Can you work these out from the drawing? Everything is in mm from the part's minimum corner. Coordinates: 2 decimals unless noted, no trailing zeros. Order: outer loops, then holes, each group sorted by start corner. A loop starts at its lowest first (then second) coordinate and runs counter-clockwise, first axis right, second up. Notation, with made-up numbers: M 83.25,84.5 L 115.25,84.5 A20 ccw 115.25,108.5 Z; hole C 68,13.5 d4. An arc over 180 degrees is marked long. Answer as CSV lines item,"result". Start each with the question number.
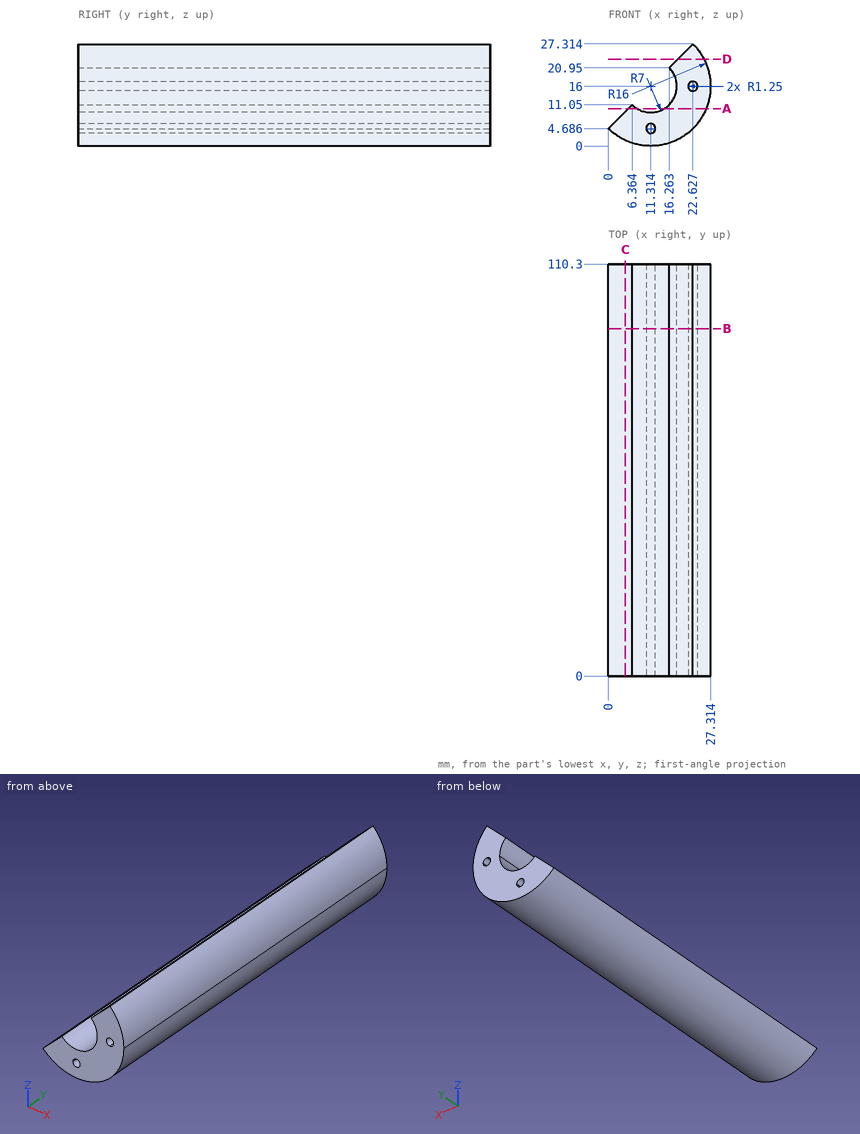
1) Suppose I cut it at D-D on z = 23.25. Please give me the cut outline in (x, y).
2) Suppose I cut it at A-A on z = 10. Please give me the cut outline in (x, y), plus the area to 3 significant figures.
3) Suppose I cut it at B-B on y = 93. Give the number of separate pieces and of enclosed holes in the cut face, plus the area to 3 significant figures.
4) Will these pins go through, and if not, where does the flat tip stop? pin 1 Ø12 at (x, z) = (23, 12) entering from -Y; pin 2 Ø12 at (x, y) = (18.5, 93) entering from -Z; pin 3 Ø8 at (y, z) = (28.5, 11.5) entering from -X (1 decimal); pin 4 Ø10 at (x, y) = (13.5, 29.5) entering from +Z (1 decimal).
5) Suppose I cut it at C-C on x = 4.5. Please give me the cut outline in (y, z), plus the area to 3 significant figures.
6) I need wall thicknesses on line 1 (Z direction, x = 22.75, y = 92.5) (1 decimal); line 2 (X direction, y = 38, z = 10.25) (1 decimal); line 3 (X direction, y = 77.5, z = 4.75) (1 decimal). Which ranges of each line are inside material? Lowest first, please. Write a range as [from, to].
Output:
1,outline,"M 18.56,0 L 25.58,0 L 25.58,110.3 L 18.56,110.3 Z"
2,outline,"M 5.31,0 L 7.71,0 L 7.71,110.3 L 5.31,110.3 Z; M 14.92,0 L 26.15,0 L 26.15,110.3 L 14.92,110.3 Z"
2,area,"1,500 mm²"
3,separate pieces,"1"
3,enclosed holes,"2"
3,area,"315 mm²"
4,pin 1,"y = 0"
4,pin 2,"z = 0.04"
4,pin 3,"x = 2.8"
4,pin 4,"z = 23.2"
5,outline,"M 0,1.52 L 110.3,1.52 L 110.3,9.19 L 0,9.19 Z"
5,area,"845 mm²"
6,line 1,"[4.8, 14.8], [17.2, 27.2]"
6,line 2,"[5.6, 7.3], [15.3, 26.2]"
6,line 3,"[0.1, 10.1], [12.6, 22.7]"
